```python
from build123d import *

# Parameters (mm, degrees)
F2_R = 1


# Not quite as in the source:
# - a fillet or chamfer that OpenCascade refuses, or shapes differently, is made with other operations: its cross-section is extruded or revolved along the edge and cut away or added


with BuildPart() as f1:
    # F0 (on Front) → F1 (revolve)
    with BuildSketch(Plane.XZ):
        with BuildLine():
            Line((0, 6.9830484122), (0, 0))
            Line((0, 0), (4.05, 0))
            Line((4.05, 0), (4.05, 3))
            Line((4.05, 3), (5.25, 3))
            Line((5.25, 3), (11, 5))
            Line((11, 5), (11, 8))
            ThreePointArc((11, 8), (5.5234543207, 7.2378272446), (0, 6.9830484122))
        make_face()
    revolve(axis=Axis((0, 0, 1.772551451), (0, 0, 1)))

    # F2
    f2_edges = [f1.edges().sort_by_distance(p)[0] for p in [
        (-11, 0, 5),
        (-11, 0, 8),
    ]]
    fillet(f2_edges, radius=F2_R)

    # F3: chamfer of 0.3 x 1.5 on 1 edges, made by hand

    # F3_s1 → F3_t2 (revolve, cut)
    with BuildSketch(Plane.XZ):
        Polygon((4.05, 1.5), (3.75, 0), (4.05, 0), align=None)
    revolve(axis=Axis((0, 0, 0), (0, 0, 1)), mode=Mode.SUBTRACT)


solid = f1.part
```
Part model, mm, in its own coordinate system. A direction names the side the tool comes from. Coordinates: 2 decimals unless noted, no trailing zeros. Order: outer loops, then holes, each group sorted by start corner. A loop starts at its lowest first (then second) coordinate and runs counter-clockwise, first axis right, second up. Notation, with made-up numbers: (26.25, 44) - (42.25, 44) arc R14 ccw to (42.25, 52) - close; hole circle Ø11 at (33.25, 3.5). An arc over 180 degrees is marked (long way). Return JSON: item names as keys, results as strings. Group by question number.
Item 1: Drill centre lines: probe 1 along Y at (x, z) = (5, 5.25); probe 2 along Y at (x, z) = (-1.25, 0.5); probe 3 along Z at (x, y) = (4.25, 9.25). Where is each one in solid material? Low to high. Write a range as from..to.
Item 2: Pin check, flat tips, straight feed: pin 1 (3 mm diameter, centred on x = -0.5, y = 5, fed in from +Z); pin 2 (3 mm diameter, centred on x = 6.5, y = -8, fed in from -Z); pin 3 (1 mm diameter, centred on y = 2, z = 5.5, fed in from -X). Stop position of each tip, or through.
Item 3: Cut at A-A (z = 1). List the corners of the cut face in (x, y), plus the area to 3 significant figures.
Item 4: Which spindle directions (+Z, -Z, +X, -X, +Y, -Y) get a long thin tool onto all of the face, cutting with end or side? Do faces 1 (the face through (0, 0, 0)), 2 (the face through (-3, -3, 3)). Say none if no direction does.
Item 5: Cut at B-B (z = 4.25). List the corners of the cut face in (x, y).
Check values:
{
 "1": {"probe 1": "y = -9.67..9.67", "probe 2": "y = -3.64..3.64", "probe 3": "z = 4.71..7.79"},
 "2": {"pin 1": "stops at z = 7.34", "pin 2": "stops at z = 4.24", "pin 3": "stops at x = -10.89"},
 "3": {"outline": "circle Ø7.9 at (0, 0)", "area": "49.0 mm2"},
 "4": {"face 1": "-Z, +X, -X, +Y, -Y", "face 2": "-Z"},
 "5": {"outline": "circle Ø17.69 at (0, 0)"}
}
